Can you work these out from the model? Positions are in its coordinate system, mm. Face numbers are marked on the shaded views. A direction names the side the tool comes from. Round coordinates to 2 decimals unless told otherwise and drop trailing zeros. Loops run counter-clockwise (first coordinate to the right, second up) from the corner with the lowest first, then second, coordinate; pieces in that order, holes last. Notation, with made-up numbers: (53, 55.5) -> (112, 55.5) arc R20 cw to (112, 75.5) -> close; hole circle Ø9 at (83.5, 3). An arc over 180 degrees is marked (long way). Write each question's results on one line, items separated by ' | '.
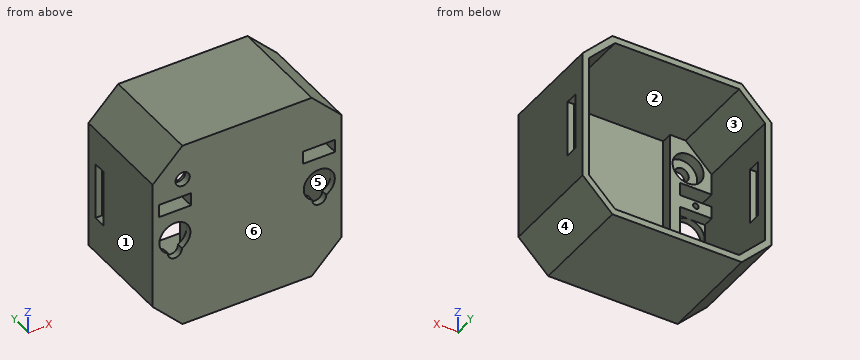
from build123d import *

# Parameters (mm, degrees)
SALIENTE_EXTRUIR1_DEPTH = 40
VACIADO1_T              = -2.5
CROQUIS5_W              = 22
CROQUIS5_H              = 5
CORTAR_EXTRUIR1_DEPTH   = 91.891418737
CORTAR_EXTRUIR2_DEPTH   = 10
SALIENTE_EXTRUIR4_DEPTH = 4.2
CROQUIS9_W              = 12.3
CROQUIS9_H              = 5
CORTAR_EXTRUIR3_DEPTH   = 64.802429421
CROQUIS10_R             = 6
CORTAR_EXTRUIR4_DEPTH   = 4
CROQUIS11_R             = 2.75
CORTAR_EXTRUIR5_DEPTH   = 4
CROQUIS12_R             = 1.1
CORTAR_EXTRUIR6_DEPTH   = 6


with BuildPart() as part:
    # Croquis3 → Saliente-Extruir1 (new body)
    with BuildSketch(Plane(origin=(0, 0, 0), x_dir=(1, 0, 0), z_dir=(0, 1, 0))):
        Polygon((-25, -36.5), (25, -36.5), (36.5, -25), (36.5, 25), (25, 36.5), (-25, 36.5), (-36.5, 25), (-36.5, -25), align=None)
    extrude(amount=SALIENTE_EXTRUIR1_DEPTH)

    # Vaciado1
    vaciado1_openings = [part.faces().sort_by_distance(p)[0] for p in [
        (0, 40, 0),
    ]]
    offset(amount=VACIADO1_T, openings=vaciado1_openings, kind=Kind.INTERSECTION)

    # Croquis5 → Cortar-Extruir1 (cut, through all)
    with BuildSketch(Plane.ZY.offset(36.5)):
        with Locations((-0.05, 33.1)):
            Rectangle(CROQUIS5_W, CROQUIS5_H)
    extrude(amount=-CORTAR_EXTRUIR1_DEPTH, mode=Mode.SUBTRACT)

    # Croquis6 → Cortar-Extruir2 (cut)
    with BuildSketch(Plane.XZ):
        with BuildLine():
            ThreePointArc((-25.210387191, -5.363392857), (-27.9, 6), (-30.589612809, -5.363392857))
            ThreePointArc((-30.589612809, -5.363392857), (-27.9, -8.3), (-25.210387191, -5.363392857))
        make_face()
        with BuildLine():
            ThreePointArc((30.589612809, -5.363392857), (27.9, -8.3), (25.210387191, -5.363392857))
            ThreePointArc((25.210387191, -5.363392857), (27.9, 6), (30.589612809, -5.363392857))
        make_face()
    extrude(amount=-CORTAR_EXTRUIR2_DEPTH, mode=Mode.SUBTRACT)

    # Croquis7 → Saliente-Extruir4 (add)
    with BuildSketch(Plane(origin=(0, 2.5, 0), x_dir=(1, 0, 0), z_dir=(0, 1, 0))):
        Polygon((-21.7, 0), (-21.7, 17), (-34, 17), (-34, 21.8), (-21.7, 21.8), (-21.7, 34), (-17.9, 34), (-17.9, -34), (-21.7, -34), (-23.964466094, -34), (-34, -23.964466094), (-34, -19.8), (-34, -15.8), (-21.7, -15.8), (-21.7, -10.8), (-34, -10.8), (-34, -6), (-21.7, -6), align=None)
        Polygon((21.7, -19.8), (21.7, -34), (17.9, -34), (17.9, 34), (21.7, 34), (21.7, 21.8), (34, 21.8), (34, 17), (21.7, 17), (21.7, 0), (21.7, -6), (34, -6), (34, -10.8), (21.7, -10.8), (21.7, -15.8), (34, -15.8), (34, -19.8), align=None)
    extrude(amount=SALIENTE_EXTRUIR4_DEPTH)

    # Croquis9 → Cortar-Extruir3 (cut, through all)
    with BuildSketch(Plane(origin=(0, 2.5, 0), x_dir=(1, 0, 0), z_dir=(0, 1, 0))):
        with Locations((-27.85, -13.3)):
            Rectangle(CROQUIS9_W, CROQUIS9_H)
        with Locations((27.85, -13.3)):
            Rectangle(CROQUIS9_W, CROQUIS9_H)
    extrude(amount=-CORTAR_EXTRUIR3_DEPTH, mode=Mode.SUBTRACT)

    # Croquis10 → Cortar-Extruir4 (cut)
    with BuildSketch(Plane(origin=(0, 6.7, 0), x_dir=(1, 0, 0), z_dir=(0, 1, 0))):
        with Locations(Location((-24.9, -22.8, 0), (0, 0, 270))):
            Circle(CROQUIS10_R)
    extrude(amount=-CORTAR_EXTRUIR4_DEPTH, mode=Mode.SUBTRACT)

    # Croquis11 → Cortar-Extruir5 (cut)
    with BuildSketch(Plane(origin=(0, 2.7, 0), x_dir=(1, 0, 0), z_dir=(0, 1, 0))):
        with Locations(Location((-24.9, -22.8, 0), (0, 0, 270))):
            Circle(CROQUIS11_R)
    extrude(amount=-CORTAR_EXTRUIR5_DEPTH, mode=Mode.SUBTRACT)

    # Croquis12 → Cortar-Extruir6 (cut)
    with BuildSketch(Plane(origin=(0, 6.7, 0), x_dir=(1, 0, 0), z_dir=(0, 1, 0))):
        with Locations(Location((-27.91, 19.1, 0), (0, 0, 270))):
            Circle(CROQUIS12_R)
        with Locations(Location((-27.91, -8.7, 0), (0, 0, 270))):
            Circle(CROQUIS12_R)
        with Locations(Location((27.91, -8.7, 0), (0, 0, 90))):
            Circle(CROQUIS12_R)
        with Locations(Location((27.91, 19.1, 0), (0, 0, 90))):
            Circle(CROQUIS12_R)
    extrude(amount=-CORTAR_EXTRUIR6_DEPTH, mode=Mode.SUBTRACT)


solid = part.part
1. If we section it at D-D (x = -7): List the corners of the cut face in (y, z) for me.
Final values:
outline: (0, -36.5) -> (40, -36.5) -> (40, -34) -> (2.5, -34) -> (2.5, 34) -> (40, 34) -> (40, 36.5) -> (0, 36.5) -> close
2. Will these pins go through, and if not, where does the flat tip stop? pin 1 (4.5 mm diameter, centred on x = -30, y = 4, fed in from +Z); pin 2 (6 mm diameter, centred on x = -9, z = -7.5, fed in from +Y); pin 3 (1 mm diameter, centred on x = -18, z = -0.5, fed in from +Y).
Final values:
pin 1: z = 33.75 | pin 2: y = 2.5 | pin 3: y = 6.7
3. If we section it at B-B (z = 22.8): List the corners of the cut face in (x, y) for me.
Final values:
outline: (-36.5, 0) -> (-27.65, 0) -> (-27.65, 2.7) -> (-30.9, 2.7) -> (-30.9, 6.7) -> (-34, 6.7) -> (-34, 40) -> (-36.5, 40) -> close; (-22.15, 0) -> (36.5, 0) -> (36.5, 40) -> (34, 40) -> (34, 2.5) -> (21.7, 2.5) -> (21.7, 6.7) -> (17.9, 6.7) -> (17.9, 2.5) -> (-17.9, 2.5) -> (-17.9, 6.7) -> (-18.9, 6.7) -> (-18.9, 2.7) -> (-22.15, 2.7) -> close
4. Please list where these lines run through material, in increasing order: line 1 (X direction, y = 1.8, z = 0); line 2 (X direction, y = 5.5, z = -12.5); line 3 (X direction, y = 2, z = -19). Write a range as from..to.
Final values:
line 1: -36.5..-33.9, -21.9..21.9, 33.9..36.5 | line 2: -36.5..-34, -21.7..-17.9, 17.9..21.7, 34..36.5 | line 3: -36.5..-29.01, -26.81..26.81, 29.01..36.5
5. We'd pull the mould along X, two halves only. Please class the marked faces 3, 4, 5 and 6: pulls with the +X half, pulls with the -X half, needs draft (parallel to the pull), parting line crosses it, or undercut.
Final values:
face 3: undercut | face 4: pulls with the +X half | face 5: undercut | face 6: needs draft
6. If we section it at A-A (y = 9): List the corners of the cut face in (x, z) for me, then the cut area to 3 significant figures.
Final values:
outline: (-36.5, -25) -> (-25, -36.5) -> (25, -36.5) -> (36.5, -25) -> (36.5, 25) -> (25, 36.5) -> (-25, 36.5) -> (-36.5, 25) -> close; hole (-34, -23.96) -> (-23.96, -34) -> (23.96, -34) -> (34, -23.96) -> (34, 23.96) -> (23.96, 34) -> (-23.96, 34) -> (-34, 23.96) -> close | area: 642 mm2
7. On a 3-axis mill with a long thin cutter (end or side, diameter ignored), from which of +Z, -Z, +X, -X, +Y, -Y can I reach the whole of each face in a straight line? I mean the marked faces 1 and 2. Say none if no direction works.
Final values:
face 1: +Z, -Z, -X, +Y, -Y | face 2: +Y
8. If we section it at C-C (z = 0): State how many separate pieces and enclosed holes the cut face has, then the cut area to 3 significant figures.
Final values:
separate pieces: 5 | enclosed holes: 0 | area: 317 mm2
